Work out the finished part from the listing and answer in its coordinate system (mm). A direction names the side the tool comes from. Round coordinates to 2 decimals unless told otherwise and drop trailing zeros. Loops run counter-clockwise (first coordinate to the right, second up) from the corner with the lowest first, then second, coordinate; pieces in that order, holes last. Notation, with made-up numbers: (4, 34) - (43, 34) arc R5 cw to (43, 38) - close; hole circle Ø4 at (-3, 68.25). An arc over 180 degrees is marked (long way). Use CSV: the item, a comma, the result in double quotes. Start each with the question number.
from build123d import *

# Parameters (mm, degrees)
SKETCH1_W           = 1041.4
SKETCH1_H           = 927.1
BOSS_EXTRUDE1_DEPTH = 508
SKETCH3_R           = 57.15
BOSS_EXTRUDE2_DEPTH = 25.4
SKETCH4_R           = 57.15
BOSS_EXTRUDE3_DEPTH = 25.4
SKETCH5_W           = 990.6
SKETCH5_H           = 876.3
CUT_EXTRUDE1_DEPTH  = 482.6
SKETCH6_R           = 50.8
CUT_EXTRUDE2_DEPTH  = 127
SKETCH7_R           = 50.8
CUT_EXTRUDE3_DEPTH  = 127
SKETCH8_W           = 927.1
SKETCH8_H           = 127
CUT_EXTRUDE4_DEPTH  = 1041.4


with BuildPart() as part:
    # Sketch1 → Boss-Extrude1 (new body)
    with BuildSketch(Plane(origin=(0, 0, 0), x_dir=(1, 0, 0), z_dir=(0, 1, 0))):
        with Locations((520.7, 463.55)):
            Rectangle(SKETCH1_W, SKETCH1_H)
    extrude(amount=BOSS_EXTRUDE1_DEPTH)

    # Sketch3 → Boss-Extrude2 (add)
    with BuildSketch(Plane.XY):
        with Locations(Location((101.6, 101.6, 0), (0, 0, 180))):
            Circle(SKETCH3_R)
        with Locations(Location((381, 101.6, 0), (0, 0, 180))):
            Circle(SKETCH3_R)
        with Locations(Location((660.4, 101.6, 0), (0, 0, 180))):
            Circle(SKETCH3_R)
        with Locations(Location((939.8, 101.6, 0), (0, 0, 180))):
            Circle(SKETCH3_R)
    extrude(amount=BOSS_EXTRUDE2_DEPTH)

    # Sketch4 → Boss-Extrude3 (add)
    with BuildSketch(Plane(origin=(0, 0, -927.1), x_dir=(-1, 0, 0), z_dir=(0, 0, -1))):
        with Locations(Location((-508, 101.6, 0), (0, 0, 180))):
            Circle(SKETCH4_R)
    extrude(amount=BOSS_EXTRUDE3_DEPTH)

    # Sketch5 → Cut-Extrude1 (cut)
    with BuildSketch(Plane(origin=(0, 508, 0), x_dir=(1, 0, 0), z_dir=(0, 1, 0))):
        with Locations((520.7, 463.55)):
            Rectangle(SKETCH5_W, SKETCH5_H)
    extrude(amount=-CUT_EXTRUDE1_DEPTH, mode=Mode.SUBTRACT)

    # Sketch6 → Cut-Extrude2 (cut)
    with BuildSketch(Plane.XY.offset(25.4)):
        with Locations((101.6, 101.6)):
            Circle(SKETCH6_R)
        with Locations((381, 101.6)):
            Circle(SKETCH6_R)
        with Locations((660.4, 101.6)):
            Circle(SKETCH6_R)
        with Locations((939.8, 101.6)):
            Circle(SKETCH6_R)
    extrude(amount=-CUT_EXTRUDE2_DEPTH, mode=Mode.SUBTRACT)

    # Sketch7 → Cut-Extrude3 (cut)
    with BuildSketch(Plane(origin=(0, 0, -952.5), x_dir=(-1, 0, 0), z_dir=(0, 0, -1))):
        with Locations((-508, 101.6)):
            Circle(SKETCH7_R)
    extrude(amount=-CUT_EXTRUDE3_DEPTH, mode=Mode.SUBTRACT)

    # Sketch8 → Cut-Extrude4 (cut)
    with BuildSketch(Plane.ZY):
        with Locations((-463.55, 444.5)):
            Rectangle(SKETCH8_W, SKETCH8_H)
    extrude(amount=-CUT_EXTRUDE4_DEPTH, mode=Mode.SUBTRACT)


solid = part.part
Item 1: A cutting plane is placed at C-C (z = -148.5). Determine the outline of the cut face in (x, y), plus the area to 3 significant figures.
Item 2: A cutting plane is placed at A-A (x = 508). Determine the outline of the cut face in (y, z).
Item 3: A cutting plane is placed at D-D (x = 850.5). Determine the outline of the cut face in (y, z).
Item 4: A cutting plane is placed at B-B (y = 252.5). Determine the outline of the cut face in (x, z).
Item 5: Which of the six approach directions +Z, -Z, +X, -X, +Y, -Y give full straight-line access (tool end or side, diameter ignored) to faces 1 (the cylindrical face through (538.72, 53.41, -939.62)), 2 (the cylindrical face through (64.158, 135.933, 0.356)), 3 (the flat face through (514, 206, -25.4))?
Item 6: Each of these flat-tipped pins is pushed along its axis until it touches: pin 1 Ø10 at (x, z) = (774, -834.5) entering from +Y; pin 2 Ø10 at (x, y) = (554, 314.5) entering from +Z. Where does it stop, or does it pass through?
Item 7: Find the intervals of material crossed by probe 1 along X at (y, z) = (101, -11); probe 2 along X at (y, z) = (347, -660); probe 3 along Y at (x, z) = (508, -927), in increasing order. Write a range as [from, to].
Item 8: The mould has two halves that part along Y. Classify faces 4 (the cylindrical face through (109.04, 44.936, 12.522)), 5 (the flat face through (514, 206, -901.7)), 6 (the cylindrical face through (545.442, 135.933, -927.456)): pulls with the +Y half, pulls with the -Y half, needs draft (parallel to the pull), parting line crosses it, or undercut.
Result sheet:
1,outline,"(0, 0) - (1041.4, 0) - (1041.4, 381) - (1016, 381) - (1016, 25.4) - (25.4, 25.4) - (25.4, 381) - (0, 381) - close"
1,area,"44,500 mm^2"
2,outline,"(0, -927.1) - (44.45, -927.1) - (44.45, -952.5) - (50.8, -952.5) - (50.8, -901.7) - (25.4, -901.7) - (25.4, -25.4) - (381, -25.4) - (381, 0) - (0, 0) - close; (152.4, -952.5) - (158.75, -952.5) - (158.75, -927.1) - (381, -927.1) - (381, -901.7) - (152.4, -901.7) - close"
3,outline,"(0, -927.1) - (381, -927.1) - (381, -901.7) - (25.4, -901.7) - (25.4, -25.4) - (381, -25.4) - (381, 0) - (0, 0) - close"
4,outline,"(0, -927.1) - (1041.4, -927.1) - (1041.4, 0) - (0, 0) - close; hole (25.4, -901.7) - (1016, -901.7) - (1016, -25.4) - (25.4, -25.4) - close"
5,face 1,"-Z"
5,face 2,"+Z"
5,face 3,"+Y"
6,pin 1,"y = 25.4"
6,pin 2,"z = 0"
7,probe 1,"[0, 50.8], [152.4, 330.2], [431.8, 609.6], [711.2, 889], [990.6, 1041.4]"
7,probe 2,"[0, 25.4], [1016, 1041.4]"
7,probe 3,"[0, 50.8], [152.4, 381]"
8,face 4,"parting line crosses it"
8,face 5,"needs draft"
8,face 6,"undercut"
